from build123d import *

# Parameters (mm, degrees)
AUFSATZ_LINEAR_AUSTRAGEN1_DEPTH = 134.46
SKIZZE3_R                       = 1
AUFSATZ_LINEAR_AUSTRAGEN2_DEPTH = 1
AUFSATZ_LINEAR_AUSTRAGEN2_TAPER = 25
LINEARES_MUSTER2_COUNT          = 12
LINEARES_MUSTER2_PITCH          = 12


with BuildPart() as part:
    # Skizze1 → Aufsatz-Linear austragen1 (new body)
    with BuildSketch(Plane(origin=(0, 0, 0), x_dir=(0, 0, -1), z_dir=(1, 0, 0))):
        with BuildLine():
            Line((-4.330127019, 2.5), (4.330127019, 2.5))
            ThreePointArc((4.330127019, 2.5), (0, -5), (-4.330127019, 2.5))
        make_face()
    extrude(amount=AUFSATZ_LINEAR_AUSTRAGEN1_DEPTH)

    # Skizze3 → Aufsatz-Linear austragen2 (add)
    with BuildSketch(Plane(origin=(0, 2.5, 0), x_dir=(1, 0, 0), z_dir=(0, 1, 0))):
        with Locations((1.229, 0)):
            Circle(SKIZZE3_R)
    aufsatz_linear_austragen2 = extrude(amount=AUFSATZ_LINEAR_AUSTRAGEN2_DEPTH, taper=AUFSATZ_LINEAR_AUSTRAGEN2_TAPER)

    # Lineares Muster2: Aufsatz-Linear austragen2 ×12
    with Locations(*[(i * LINEARES_MUSTER2_PITCH, 0, 0) for i in range(1, LINEARES_MUSTER2_COUNT)]):
        add(aufsatz_linear_austragen2)


solid = part.part
The listing builds one solid part. Answer for the finished solid, in the listing's coordinates (mm). Round coordinates to 2 decimals unless told otherwise and drop trailing zeros. Order: outer loops, then holes, each group sorted by start corner. A loop starts at its lowest first (then second) coordinate and runs counter-clockwise, first axis right, second up. Notation, with made-up numbers: (89, 12.5) -> (94, 12.5) arc R18 cw to (94, 30.5) -> close; hole circle Ø1 at (49.5, -23.5). An arc over 180 degrees is marked (long way). Write each question's results on one line, items separated by ' | '. Start each with the question number.
Q1. The mould has two halves that part along X. Classify faces 1 (the flat face through (134.46, 0, 0)), 2 (the cylindrical face through (66, -5, 0)), 3 (the flat face through (66, 2.5, 0)), 4 (the flat face through (0, 0, 0)): pulls with the +X half, pulls with the -X half, needs draft (parallel to the pull), parting line crosses it, or undercut.
Q2. Each of these flat-tipped pins is pushed along its axis until it touches: pin 1 (2 mm diameter, centred on y = -3.5, z = -1.5, fed in from -X); pin 2 (2 mm diameter, centred on x = 54, z = 2, fed in from -Y). Where does it stop, or does it pass through?
Q3. Find section B-B (y = -1). Determine the outline of the cut face in (x, z), then the cut area to 3 significant figures.
Q4. Find section A-A (x = 101). Determine the outline of the cut face in (y, z).
Q5. Straight lines are drawn through the part: probe 1 along Y at (x, z) = (105, 0.5); probe 2 along Y at (x, z) = (51, 1.25); probe 3 along Z at (x, y) = (90.5, -1.5). For each, find the intervals that lie inside material, in ascending order. Write a range as from..to.
Worked answers:
1) face 1: pulls with the +X half | face 2: needs draft | face 3: undercut | face 4: pulls with the -X half
2) pin 1: stops at x = 0 | pin 2: stops at y = -4.9
3) outline: (0, -4.9) -> (134.46, -4.9) -> (134.46, 4.9) -> (0, 4.9) -> close | area: 1,320 mm2
4) outline: (2.5, -4.33) -> (2.5, 4.33) arc R5 ccw (long way) to start
5) probe 1: y = -4.97..2.5 | probe 2: y = -4.84..2.5 | probe 3: z = -4.77..4.77
